```python
from build123d import *

# Parameters (mm, degrees)
SKETCH1_W                                           = 80
SKETCH1_H                                           = 225
BOSS_EXTRUDE1_DEPTH                                 = 20
CUT_EXTRUDE1_REACH                                  = 125.176
CUT_EXTRUDE2_REACH                                  = 125.176
CUT_EXTRUDE3_REACH                                  = 125.176
CUT_EXTRUDE4_REACH                                  = 125.176
CBORE_FOR_M8_HEX_SOCKET_HEAD_CAP_SCREW1_D           = 8.4
CBORE_FOR_M8_HEX_SOCKET_HEAD_CAP_SCREW1_CBORE_D     = 15
CBORE_FOR_M8_HEX_SOCKET_HEAD_CAP_SCREW1_CBORE_DEPTH = 8.6
F_8_0MM_DOWEL_HOLE1_D                               = 8
CUT_EXTRUDE5_REACH                                  = 125.176
SKETCH7_R                                           = 10


with BuildPart() as part:
    # Sketch1 → Boss-Extrude1 (new body)
    with BuildSketch(Plane(origin=(0, 0, 0), x_dir=(1, 0, 0), z_dir=(0, 1, 0))):
        with Locations((-6, 0)):
            Rectangle(SKETCH1_W, SKETCH1_H)
    extrude(amount=-BOSS_EXTRUDE1_DEPTH)

    # Sketch2 → Cut-Extrude1 (cut, up to next)
    with BuildSketch(Plane(origin=(0, 0, 0), x_dir=(1, 0, 0), z_dir=(0, 1, 0)), mode=Mode.PRIVATE) as cut_extrude1_sk1:
        with BuildLine():
            Line((21, -19.64), (29.5, -19.64))
            ThreePointArc((29.5, -19.64), (30.207106781, -19.347106781), (30.5, -18.64))
            Line((30.5, -18.64), (30.5, 23.36))
            ThreePointArc((30.5, 23.36), (30.207106781, 24.067106781), (29.5, 24.36))
            Line((29.5, 24.36), (21, 24.36))
            ThreePointArc((21, 24.36), (20.292893219, 24.067106781), (20, 23.36))
            Line((20, 23.36), (20, -18.64))
            ThreePointArc((20, -18.64), (20.292893219, -19.347106781), (21, -19.64))
        make_face()
    cut_extrude1_tool1 = extrude(cut_extrude1_sk1.sketch, amount=-CUT_EXTRUDE1_REACH, mode=Mode.PRIVATE) & part.part
    add(cut_extrude1_tool1.solids().sort_by_distance((25.25, 0, -2.36))[0], mode=Mode.SUBTRACT)

    # Sketch4 → Cut-Extrude2 (cut, up to next)
    with BuildSketch(Plane(origin=(0, 0, 0), x_dir=(1, 0, 0), z_dir=(0, 1, 0)), mode=Mode.PRIVATE) as cut_extrude2_sk1:
        with BuildLine():
            Line((7, -68.64), (7, -45.14))
            Line((7, -45.14), (-7, -45.14))
            Line((-7, -45.14), (-7, -68.64))
            ThreePointArc((-7, -68.64), (-6.707106781, -69.347106781), (-6, -69.64))
            Line((-6, -69.64), (6, -69.64))
            ThreePointArc((6, -69.64), (6.707106781, -69.347106781), (7, -68.64))
        make_face()
    cut_extrude2_tool1 = extrude(cut_extrude2_sk1.sketch, amount=-CUT_EXTRUDE2_REACH, mode=Mode.PRIVATE) & part.part
    add(cut_extrude2_tool1.solids().sort_by_distance((0, 0, 57.374932))[0], mode=Mode.SUBTRACT)

    # Sketch5 → Cut-Extrude3 (cut, up to next)
    with BuildSketch(Plane(origin=(0, 0, 0), x_dir=(1, 0, 0), z_dir=(0, 1, 0)), mode=Mode.PRIVATE) as cut_extrude3_sk1:
        with BuildLine():
            Line((-18.5, -13.64), (-18.5, 33.36))
            Line((-18.5, 33.36), (-40.5, 33.36))
            ThreePointArc((-40.5, 33.36), (-41.207106781, 33.067106781), (-41.5, 32.36))
            Line((-41.5, 32.36), (-41.5, -12.64))
            ThreePointArc((-41.5, -12.64), (-41.207106781, -13.347106781), (-40.5, -13.64))
            Line((-40.5, -13.64), (-18.5, -13.64))
        make_face()
    cut_extrude3_tool1 = extrude(cut_extrude3_sk1.sketch, amount=-CUT_EXTRUDE3_REACH, mode=Mode.PRIVATE) & part.part
    add(cut_extrude3_tool1.solids().sort_by_distance((-29.995521, 0, -9.86))[0], mode=Mode.SUBTRACT)

    # Sketch6 → Cut-Extrude4 (cut, up to next)
    with BuildSketch(Plane(origin=(0, 0, 0), x_dir=(1, 0, 0), z_dir=(0, 1, 0)), mode=Mode.PRIVATE) as cut_extrude4_sk1:
        with BuildLine():
            Line((19, 69.64), (-19, 69.64))
            ThreePointArc((-19, 69.64), (-19.707106781, 69.347106781), (-20, 68.64))
            Line((-20, 68.64), (-20, 53.36))
            Line((-20, 53.36), (20, 53.36))
            Line((20, 53.36), (20, 68.64))
            ThreePointArc((20, 68.64), (19.707106781, 69.347106781), (19, 69.64))
        make_face()
    cut_extrude4_tool1 = extrude(cut_extrude4_sk1.sketch, amount=-CUT_EXTRUDE4_REACH, mode=Mode.PRIVATE) & part.part
    add(cut_extrude4_tool1.solids().sort_by_distance((0, 0, -61.494779))[0], mode=Mode.SUBTRACT)

    # CBORE for M8 Hex Socket Head Cap Screw1 (through all)
    with Locations(Plane(origin=(0, -20, 0), x_dir=(-1, 0, 0), z_dir=(0, -1, 0))):
        with Locations((-19, 102.5), (31, 102.5), (-19, -102.5), (31, -102.5)):
            CounterBoreHole(CBORE_FOR_M8_HEX_SOCKET_HEAD_CAP_SCREW1_D / 2, CBORE_FOR_M8_HEX_SOCKET_HEAD_CAP_SCREW1_CBORE_D / 2, CBORE_FOR_M8_HEX_SOCKET_HEAD_CAP_SCREW1_CBORE_DEPTH)

    # Ø8.0mm Dowel Hole1 (through all)
    with Locations(Plane(origin=(0, -20, 0), x_dir=(-1, 0, 0), z_dir=(0, -1, 0))):
        with Locations((-3.5, 102.5), (15.5, -102.5)):
            Hole(F_8_0MM_DOWEL_HOLE1_D / 2)

    # Sketch7 → Cut-Extrude5 (cut, up to next)
    with BuildSketch(Plane(origin=(0, 0, 0), x_dir=(1, 0, 0), z_dir=(0, 1, 0)), mode=Mode.PRIVATE) as cut_extrude5_sk1:
        with Locations(Location((-31, -33, 0), (0, 0, 270))):
            Circle(SKETCH7_R)
    cut_extrude5_tool1 = extrude(cut_extrude5_sk1.sketch, amount=-CUT_EXTRUDE5_REACH, mode=Mode.PRIVATE) & part.part
    # Sketch7 → Cut-Extrude5 (cut, up to next)
    with BuildSketch(Plane(origin=(0, 0, 0), x_dir=(1, 0, 0), z_dir=(0, 1, 0)), mode=Mode.PRIVATE) as cut_extrude5_sk2:
        with Locations(Location((-6, 82.5, 0), (0, 0, 270))):
            Circle(SKETCH7_R)
    cut_extrude5_tool2 = extrude(cut_extrude5_sk2.sketch, amount=-CUT_EXTRUDE5_REACH, mode=Mode.PRIVATE) & part.part
    # Sketch7 → Cut-Extrude5 (cut, up to next)
    with BuildSketch(Plane(origin=(0, 0, 0), x_dir=(1, 0, 0), z_dir=(0, 1, 0)), mode=Mode.PRIVATE) as cut_extrude5_sk3:
        with Locations(Location((19, -33, 0), (0, 0, 270))):
            Circle(SKETCH7_R)
    cut_extrude5_tool3 = extrude(cut_extrude5_sk3.sketch, amount=-CUT_EXTRUDE5_REACH, mode=Mode.PRIVATE) & part.part
    # Sketch7 → Cut-Extrude5 (cut, up to next)
    with BuildSketch(Plane(origin=(0, 0, 0), x_dir=(1, 0, 0), z_dir=(0, 1, 0)), mode=Mode.PRIVATE) as cut_extrude5_sk4:
        with Locations(Location((-31, 47, 0), (0, 0, 270))):
            Circle(SKETCH7_R)
    cut_extrude5_tool4 = extrude(cut_extrude5_sk4.sketch, amount=-CUT_EXTRUDE5_REACH, mode=Mode.PRIVATE) & part.part
    # Sketch7 → Cut-Extrude5 (cut, up to next)
    with BuildSketch(Plane(origin=(0, 0, 0), x_dir=(1, 0, 0), z_dir=(0, 1, 0)), mode=Mode.PRIVATE) as cut_extrude5_sk5:
        with Locations(Location((19, 39, 0), (0, 0, 270))):
            Circle(SKETCH7_R)
    cut_extrude5_tool5 = extrude(cut_extrude5_sk5.sketch, amount=-CUT_EXTRUDE5_REACH, mode=Mode.PRIVATE) & part.part
    # Sketch7 → Cut-Extrude5 (cut, up to next)
    with BuildSketch(Plane(origin=(0, 0, 0), x_dir=(1, 0, 0), z_dir=(0, 1, 0)), mode=Mode.PRIVATE) as cut_extrude5_sk6:
        with Locations(Location((-31, -82.5, 0), (0, 0, 270))):
            Circle(SKETCH7_R)
    cut_extrude5_tool6 = extrude(cut_extrude5_sk6.sketch, amount=-CUT_EXTRUDE5_REACH, mode=Mode.PRIVATE) & part.part
    # Sketch7 → Cut-Extrude5 (cut, up to next)
    with BuildSketch(Plane(origin=(0, 0, 0), x_dir=(1, 0, 0), z_dir=(0, 1, 0)), mode=Mode.PRIVATE) as cut_extrude5_sk7:
        with Locations(Location((-6, -82.5, 0), (0, 0, 270))):
            Circle(SKETCH7_R)
    cut_extrude5_tool7 = extrude(cut_extrude5_sk7.sketch, amount=-CUT_EXTRUDE5_REACH, mode=Mode.PRIVATE) & part.part
    # Sketch7 → Cut-Extrude5 (cut, up to next)
    with BuildSketch(Plane(origin=(0, 0, 0), x_dir=(1, 0, 0), z_dir=(0, 1, 0)), mode=Mode.PRIVATE) as cut_extrude5_sk8:
        with Locations(Location((19, -82.5, 0), (0, 0, 270))):
            Circle(SKETCH7_R)
    cut_extrude5_tool8 = extrude(cut_extrude5_sk8.sketch, amount=-CUT_EXTRUDE5_REACH, mode=Mode.PRIVATE) & part.part
    # Sketch7 → Cut-Extrude5 (cut, up to next)
    with BuildSketch(Plane(origin=(0, 0, 0), x_dir=(1, 0, 0), z_dir=(0, 1, 0)), mode=Mode.PRIVATE) as cut_extrude5_sk9:
        with Locations(Location((-31, 82.5, 0), (0, 0, 270))):
            Circle(SKETCH7_R)
    cut_extrude5_tool9 = extrude(cut_extrude5_sk9.sketch, amount=-CUT_EXTRUDE5_REACH, mode=Mode.PRIVATE) & part.part
    # Sketch7 → Cut-Extrude5 (cut, up to next)
    with BuildSketch(Plane(origin=(0, 0, 0), x_dir=(1, 0, 0), z_dir=(0, 1, 0)), mode=Mode.PRIVATE) as cut_extrude5_sk10:
        with Locations(Location((19, 82.5, 0), (0, 0, 270))):
            Circle(SKETCH7_R)
    cut_extrude5_tool10 = extrude(cut_extrude5_sk10.sketch, amount=-CUT_EXTRUDE5_REACH, mode=Mode.PRIVATE) & part.part
    add(cut_extrude5_tool1.solids().sort_by_distance((-31, 0, 33))[0], mode=Mode.SUBTRACT)
    add(cut_extrude5_tool2.solids().sort_by_distance((-6, 0, -82.5))[0], mode=Mode.SUBTRACT)
    add(cut_extrude5_tool3.solids().sort_by_distance((19, 0, 33))[0], mode=Mode.SUBTRACT)
    add(cut_extrude5_tool4.solids().sort_by_distance((-31, 0, -47))[0], mode=Mode.SUBTRACT)
    add(cut_extrude5_tool5.solids().sort_by_distance((19, 0, -39))[0], mode=Mode.SUBTRACT)
    add(cut_extrude5_tool6.solids().sort_by_distance((-31, 0, 82.5))[0], mode=Mode.SUBTRACT)
    add(cut_extrude5_tool7.solids().sort_by_distance((-6, 0, 82.5))[0], mode=Mode.SUBTRACT)
    add(cut_extrude5_tool8.solids().sort_by_distance((19, 0, 82.5))[0], mode=Mode.SUBTRACT)
    add(cut_extrude5_tool9.solids().sort_by_distance((-31, 0, -82.5))[0], mode=Mode.SUBTRACT)
    add(cut_extrude5_tool10.solids().sort_by_distance((19, 0, -82.5))[0], mode=Mode.SUBTRACT)


solid = part.part
```
Build history of the part. All positions in model axes, mm. A direction names the side the tool comes from. Round coordinates to 2 decimals unless told otherwise and drop trailing zeros. Loops run counter-clockwise (first coordinate to the right, second up) from the corner with the lowest first, then second, coordinate; pieces in that order, holes last. Notation, with made-up numbers: M 1.25,-25.5 L 59.25,-25.5 A18 ccw 59.25,-20.5 Z; hole C 55.5,53.5 d9. An arc over 180 degrees is marked long. Answer as CSV lines item,"result".
1. Flat gauge pins, fed straight in: P1, Ø9, axis at x = 19, z = -102.5, coming from the -Y side; P2, Ø6.5, axis at x = -15.5, z = 102.5, coming from the +Y side. Where does each tip first touch, or does it go through?
Resolved:
P1,"stops at y = -11.4"
P2,"passes through"
2. 3-axis set-ups, long thin cutter, end or side, ignore diameter. For faces 3 (the flat face through (0, -10, -69.64)), 4 (the flat face through (-34, -11.4, 106)): which of +Z, -Z, +X, -X, +Y, -Y reach the whole face in a straight line?
Resolved:
face 3,"+Y, -Y"
face 4,"-Y"
3. Two-plate mould, pull along X, no slides. Class faces 1 (the cylindrical face through (-37, -10, -55)), 2 (the flat face through (-46, -10, 2)): released by +X, released by -X, zero draft, split by the parting line, or undercut.
Resolved:
face 1,"undercut"
face 2,"released by -X"
4. Cut at B-B on z = -47. Write the cut outline in (x, y).
Resolved:
outline,"M -46,-20 L -41,-20 L -41,0 L -46,0 Z; M -21,-20 L 13,-20 L 13,0 L -21,0 Z; M 25,-20 L 34,-20 L 34,0 L 25,0 Z"
5. Wall check: probe 1 along X at (y, z) = (-11, 82.5); probe 2 along X at (y, z) = (-8.5, -102.5); probe 3 along X at (y, z) = (-7, 64). Give the ranges that are in metal, low to high. Write a range as [from, to].
Resolved:
probe 1,"x = [-46, -41], [-21, -16], [4, 9], [29, 34]"
probe 2,"x = [-46, -35.2], [-26.8, -0.5], [7.5, 14.8], [23.2, 34]"
probe 3,"x = [-46, -7], [7, 34]"
6. Cut at D-D on x = 1.5. Write the cut outline in (y, z), then the cut area to 3 significant figures.
Resolved:
outline,"M -20,-112.5 L 0,-112.5 L 0,-105.96 L -20,-105.96 Z; M -20,-99.04 L 0,-99.04 L 0,-89.11 L -20,-89.11 Z; M -20,-75.89 L 0,-75.89 L 0,-69.64 L -20,-69.64 Z; M -20,-53.36 L 0,-53.36 L 0,45.14 L -20,45.14 Z; M -20,69.64 L 0,69.64 L 0,75.89 L -20,75.89 Z; M -20,89.11 L 0,89.11 L 0,112.5 L -20,112.5 Z"
area,"3,020 mm²"
7. Cut at A-A on z = 102.5. Write the cut outline in (x, y).
Resolved:
outline,"M -46,-20 L -38.5,-20 L -38.5,-11.4 L -35.2,-11.4 L -35.2,0 L -46,0 Z; M -26.8,-11.4 L -23.5,-11.4 L -23.5,-20 L -19.5,-20 L -19.5,0 L -26.8,0 Z; M -11.5,-20 L 11.5,-20 L 11.5,-11.4 L 14.8,-11.4 L 14.8,0 L -11.5,0 Z; M 23.2,-11.4 L 26.5,-11.4 L 26.5,-20 L 34,-20 L 34,0 L 23.2,0 Z"
8. Cut at C-C on y = -2.75. Count the separate pieces of the cut face and the enclosed holes in it, then the cut area to 3 significant figures.
Resolved:
separate pieces,"1"
enclosed holes,"20"
area,"12,000 mm²"
